Input: part model. Units: mm. Frame: model coordinates. A direction names the side the tool comes from. Round coordinates to 2 decimals unless told otherwise and drop trailing zeros. Write each loop counter-clockwise with the first axis right and the second up, starting at its lowest first coordinate (ties: lowest second). Pieces come first, ordered by that corner, then holes. Notation, with made-up numbers: (59, -39.5) -> (106, -39.5) arc R22 cw to (106, -13.5) -> close; hole circle Ø2 at (-22.75, 35.5). An arc over 180 degrees is marked (long way). Write item = value, one per line.
Autodesk Inventor part; units mm, degrees
ref_plane "YZ Plane" through (0, 0, 0) normal (1, 0, 0) x (0, 1, 0)
ref_plane "XZ Plane" through (0, 0, 0) normal (0, 1, 0) x (-1, 0, 0)
ref_plane "XY Plane" through (0, 0, 0) normal (0, 0, 1) x (1, 0, 0)
sketch "Sketch1" plane through (0, 0, 0) normal (0, 1, 0) x (-1, 0, 0)
  line L0 (1.5, -2.15) -> (2.25, -2.15)
  line L1 (4.15, -2.96) -> (-1, -2.96)
  line L2 (-1, -2.96) -> (-1, -5)
  line L3 (0.8364, -2.3) -> (-2, -2.3)
  line L4 (-1, -5) -> (-2, -5)
  line L5 (-2, -5) -> (-2, -2.3)
  line L6 (-0.8, -0.5) -> (0.8364, -2.3)
  line L7 (0, 0) -> (-5, 0) construction
  line L8 (1.5, -2.15) -> (0, -0.5)
  line L9 (0, -0.5) -> (-0.8, -0.5)
  line L10 (2.25, -2.15) -> (3.25, -0.5)
  line L11 (3.25, -0.5) -> (4.05, -0.5)
  line L12 (4.05, -0.5) -> (4.15, -2.96)
  dimension "d0" = 2.3
  dimension "d4" = 2.15
  dimension "d5" = 0.75
  dimension "d9" = 0.81
  dimension "d10" = 1
  dimension "d11" = 5
  dimension "d22" = 0.8
  dimension "d27" = 0.8
  dimension "d45" = 3.5
  dimension "d47" = 1.5
  dimension "d48" = 0.1
  dimension "d54" = 0.5
  dimension "d55" = 1
sketch "Sketch4" plane through (0, 0, 0) normal (0, 1, 0) x (-1, 0, 0)
  line L0 (0, 1.25) -> (0, 2.85)
  line L1 (0, 2.85) -> (6.625, 2.85)
  line L2 (6.625, 2.85) -> (6.625, 1.25)
  line L3 (3.625, 0.5) -> (5.175, 2.05)
  line L4 (5.175, 2.05) -> (5.825, 2.05)
  line L5 (5.825, 2.05) -> (6.625, 1.25)
  line L6 (0, 1.25) -> (2, 1.25)
  line L7 (2, 1.25) -> (2.75, 0.5)
  line L8 (2.75, 0.5) -> (3.625, 0.5)
  line L9 (3.625, 0.5) -> (3.625, 2.85)
  line L10 (0, 0) -> (1.5, 0)
  point P0 (5.5, 2.05)
  dimension "d56" = 1.25
  dimension "d57" = 2
  dimension "d58" = 135
  dimension "d59" = 0.5
  dimension "d61" = 2.05
  dimension "d62" = 0.65
  dimension "d63" = 0.8
  dimension "d65" = 3.5
  dimension "d68" = 1.6
revolve "Revolution5" add sketch "Sketch4" angle 360 about axis through (0, 0, 0) along (-1, 0, 0) contours L0 L1 L9 L8 L7 L6
revolve "Revolution6" add sketch "Sketch4" angle 220 mid plane about axis through (0, 0, 0) along (-1, 0, 0)
sketch "Sketch5" plane through (0, 0, 0) normal (1, 0, 0) x (0, 0, -1)
  circle A0 centre (0, 0) radius 2.85
  line L0 (-0.4, 2.8218) -> (-0.4, 10.8218)
  line L1 (-0.4, 10.8218) -> (0.4, 10.8218)
  line L2 (0.4, 10.8218) -> (0.4, 2.8218)
  arc A1 (0.9748, 2.6781) -> (0.9748, -2.6781) centre (0, 0) ccw
  line L3 (-2.8218, -0.4) -> (-10.8218, -0.4)
  line L4 (-10.8218, -0.4) -> (-10.8218, 0.4)
  line L5 (-10.8218, 0.4) -> (-2.8218, 0.4)
  line L6 (-0.4, -2.8218) -> (-0.4, -10.8218)
  line L7 (-0.4, -10.8218) -> (0.4, -10.8218)
  line L8 (0.4, -10.8218) -> (0.4, -2.8218)
  point P0 (-2.8218, 0.4)
  point P1 (0.4, -2.8218)
  dimension "d69" = 0.8
  dimension "d70" = 8
  dimension "d15" = 1.2
  dimension "d30" = 1.2
  dimension "d31" = 1.2
  dimension "d34" = 3.5
  dimension "d50" = 120
  dimension "d51" = 0.8
extrude "Extrusion5" add sketch "Sketch5" against normal up to surface (6.625 mm away) contours L8 L7 L6 A0
sketch "Sketch3" plane through (-9.15, 0, 0) normal (-1, 0, 0) x (0, 1, 0)
  arc A0 (1, 0.4583) -> (0, -1.1) centre (0, 0) ccw
  arc A1 (1, 0.4583) -> (0, -1.1) centre (0, 0) ccw
  arc A2 (1.0439, -0.3469) -> (-1.0439, -0.3469) centre (0, 2.5349) ccw
  arc A3 (0.6833, -0.8621) -> (-0.6833, -0.8621) centre (0, 2.5349) ccw
  circle A4 centre (0, 0) radius 6
  dimension "d42" = 0.4
properties part number "adjustable_collimator"
1) Draft query along Z for faces 1 (the face through (-1.01, -1.22, -0.27)), 2 (the face through (-3, -7, -0.4)), 3 (the face through (0, -1.42, 0.01)), 4 (the face through (-4.066, -0.025, 0.941)). Return one class per face: +Z half, -Z half, draft (parallel to the pull), parting line (faces both ways), or undercut.
Solutions:
face_1 = undercut
face_2 = -Z half
face_3 = draft
face_4 = undercut
2) First-contact query: P1, Ø2, axis at y = 0, z = 0, coming from the -X side (3 decimals); P2, Ø1.5, axis at x = -1, z = -1.5, coming from the +Y side; P3, Ø1, axis at x = -4.5, y = -8.5, coming from the -Z side; P4, Ø2, axis at y = -1, z = -1, coming from the -X side (3 decimals). Flat tips, straight axial feed; report the tip coordinate or a pass-through.
Solutions:
P1 = -4.125
P2 = 2.75
P3 = -0.4
P4 = -6.625
3) Access query for faces 5 (the face through (-3.194, -0.488, -0.108)), 6 (the face through (-4.771, -2.08, -0.757)), 7 (the face through (-3, -7, 0.4)), 8 (the face through (-5.5, -0.06, 2.05)), 9 (the face through (-6.625, -2, 1)). Directions: +Z, -Z, +X, -X, +Y, -Y. A direction counts if a zero-diameter tool reaches every point of the face in a straight line with its end or side. Return the directions, or none.
Solutions:
face_5 = +X, -X
face_6 = -Z, -X
face_7 = +Z, +X, -X, -Y
face_8 = none
face_9 = +Z, -Z, -X, +Y, -Y
4) Cut plane B-B (z = 0). Return the cut outline in (x, y) (3 decimals), and give its area (3 significant figures).
Solutions:
outline = (-6.625, -10.822) -> (0, -10.822) -> (0, -1.25) -> (-2, -1.25) -> (-2.75, -0.5) -> (-3.625, -0.5) -> (-5.175, -2.05) -> (-5.825, -2.05) -> (-6.625, -1.25) -> close; (-6.625, 1.25) -> (-5.825, 2.05) -> (-5.175, 2.05) -> (-3.625, 0.5) -> (-2.75, 0.5) -> (-2, 1.25) -> (0, 1.25) -> (0, 2.85) -> (-6.625, 2.85) -> close
area = 74.1 mm^2
5) Cut plane D-D (x = -5.5). Return the cut outline in (y, z).
Solutions:
outline = (-10.82, -0.4) -> (-2.82, -0.4) arc R2.85 ccw to (-2.68, -0.97) -> (-1.93, -0.7) arc R2.05 cw (long way) to (1.93, -0.7) -> (2.68, -0.97) arc R2.85 ccw (long way) to (-2.82, 0.4) -> (-10.82, 0.4) -> close
6) Cut plane A-A (x = -2.5). Return the cut outline in (y, z).
Solutions:
outline = (-10.82, -0.4) -> (-2.82, -0.4) arc R2.85 ccw (long way) to (-2.82, 0.4) -> (-10.82, 0.4) -> close; hole circle Ø1.5 at (0, 0)
7) Line query: L1, parallel to Z at x = -5.4, y = 0; L2, parallel to Z at x = -1.5, y = -4; L3, parallel to Y at x = -5.55, z = 0. Output: solid intervals per line, ascending. Write a range as from..to.
Solutions:
L1 = 2.05..2.85
L2 = -0.4..0.4
L3 = -10.82..-2.05, 2.05..2.85
8) Cut plane C-C (y = 0). Return the cut outline in (x, z) (3 decimals), and give its area (3 significant figures).
Solutions:
outline = (-6.625, 1.25) -> (-5.825, 2.05) -> (-5.175, 2.05) -> (-3.625, 0.5) -> (-2.75, 0.5) -> (-2, 1.25) -> (0, 1.25) -> (0, 2.85) -> (-6.625, 2.85) -> close; (-3.625, -2.85) -> (0, -2.85) -> (0, -1.25) -> (-2, -1.25) -> (-2.75, -0.5) -> (-3.625, -0.5) -> close
area = 17.4 mm^2
